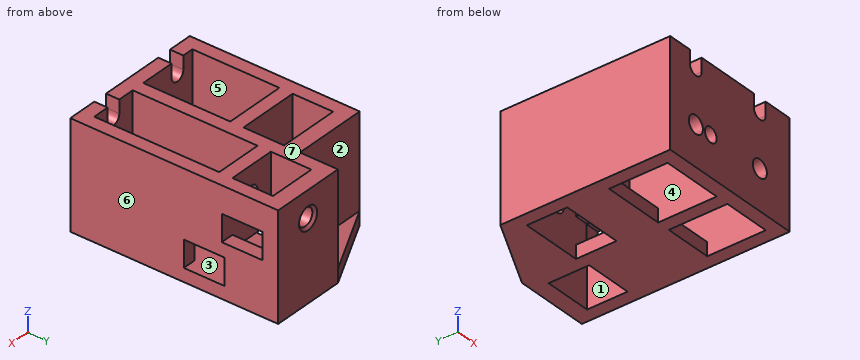
from build123d import *

# Parameters (mm, degrees)
SKETCH1_W           = 23
SKETCH1_H           = 32.75
SKETCH1_W_2         = 18
SKETCH1_H_2         = 15.25
SKETCH1_H_3         = 47.05
BOSS_EXTRUDE1_DEPTH = 40
CUT_EXTRUDE1_REACH  = 106.244
SKETCH2_R           = 2.75
CUT_EXTRUDE2_REACH  = 106.244
SKETCH3_W           = 10
SKETCH3_H           = 15.25
SKETCH4_W           = 10
SKETCH4_H           = 15.25
CUT_EXTRUDE3_DEPTH  = 102.645904984
CUT_EXTRUDE4_REACH  = 106.244
SKETCH6_R           = 3.25
CHAMFER1_SIZE       = 1
CUT_EXTRUDE5_REACH  = 106.244
SKETCH7_R           = 3.3
SKETCH9_R           = 2.75
CUT_EXTRUDE6_DEPTH  = 101.542975886
SKETCH10_W          = 18
SKETCH10_H          = 25
SKETCH10_W_2        = 23
SKETCH10_H_2        = 10.7
BOSS_EXTRUDE2_DEPTH = 5


with BuildPart() as part:
    # Sketch1 → Boss-Extrude1 (new body)
    with BuildSketch(Plane.XY):
        Polygon((0, 0), (0, 64), (28, 64), (28, 78.3), (56, 78.3), (56, 0), align=None)
        with Locations((16.5, 21.375)):
            Rectangle(SKETCH1_W, SKETCH1_H, mode=Mode.SUBTRACT)
        with Locations((42, 64.675)):
            Rectangle(SKETCH1_W_2, SKETCH1_H_2, mode=Mode.SUBTRACT)
        with Locations((16.5, 50.375)):
            Rectangle(SKETCH1_W, SKETCH1_H_2, mode=Mode.SUBTRACT)
        with Locations((42, 28.525)):
            Rectangle(SKETCH1_W_2, SKETCH1_H_3, mode=Mode.SUBTRACT)
    extrude(amount=BOSS_EXTRUDE1_DEPTH)

    # Cut-Extrude1: up to this face of the body (flat: up to its plane)
    cut_extrude1_end = Plane(part.part.faces().sort_by_distance((16.5, 37.75, 20))[0])
    # Sketch2 → Cut-Extrude1 (cut, up to the picked face)
    with BuildSketch(Plane(origin=(0, 78.3, 0), x_dir=(1, 0, 0), z_dir=(0, 1, 0)), mode=Mode.PRIVATE) as cut_extrude1_sk1:
        with Locations(Location((19, -15, 0), (0, 0, 270))):
            Circle(SKETCH2_R)
    cut_extrude1_tool1 = split(extrude(cut_extrude1_sk1.sketch, amount=-CUT_EXTRUDE1_REACH, mode=Mode.PRIVATE), bisect_by=cut_extrude1_end, keep=Keep.BOTH, mode=Mode.PRIVATE)
    # Sketch2 → Cut-Extrude1 (cut, up to the picked face)
    with BuildSketch(Plane(origin=(0, 78.3, 0), x_dir=(1, 0, 0), z_dir=(0, 1, 0)), mode=Mode.PRIVATE) as cut_extrude1_sk2:
        with Locations(Location((42, -30, 0), (0, 0, 270))):
            Circle(SKETCH2_R)
    cut_extrude1_tool2 = split(extrude(cut_extrude1_sk2.sketch, amount=-CUT_EXTRUDE1_REACH, mode=Mode.PRIVATE), bisect_by=cut_extrude1_end, keep=Keep.BOTH, mode=Mode.PRIVATE)
    add(cut_extrude1_tool1.solids().sort_by(Axis((19, 78.3, 15), (0, -1, 0)))[0], mode=Mode.SUBTRACT)
    add(cut_extrude1_tool2.solids().sort_by(Axis((42, 78.3, 30), (0, -1, 0)))[0], mode=Mode.SUBTRACT)

    # Sketch3 → Cut-Extrude2 (cut, up to next)
    with BuildSketch(Plane(origin=(56, 0, 0), x_dir=(0, 0, -1), z_dir=(1, 0, 0)), mode=Mode.PRIVATE) as cut_extrude2_sk1:
        with Locations((-25, 64.675)):
            Rectangle(SKETCH3_W, SKETCH3_H)
    cut_extrude2_tool1 = extrude(cut_extrude2_sk1.sketch, amount=-CUT_EXTRUDE2_REACH, mode=Mode.PRIVATE) & part.part
    add(cut_extrude2_tool1.solids().sort_by_distance((56, 64.675, 25))[0], mode=Mode.SUBTRACT)

    # Sketch4 → Cut-Extrude3 (cut, through all)
    with BuildSketch(Plane(origin=(5, 0, 0), x_dir=(0, 0, -1), z_dir=(1, 0, 0))):
        with Locations((-10, 50.375)):
            Rectangle(SKETCH4_W, SKETCH4_H)
    extrude(amount=CUT_EXTRUDE3_DEPTH, mode=Mode.SUBTRACT)

    # Sketch6 → Cut-Extrude4 (cut, up to next)
    with BuildSketch(Plane(origin=(0, 78.3, 0), x_dir=(1, 0, 0), z_dir=(0, 1, 0)), mode=Mode.PRIVATE) as cut_extrude4_sk1:
        with Locations(Location((19, -15, 0), (0, 0, 270))):
            Circle(SKETCH6_R)
    cut_extrude4_tool1 = extrude(cut_extrude4_sk1.sketch, amount=-CUT_EXTRUDE4_REACH, mode=Mode.PRIVATE) & part.part
    # Sketch6 → Cut-Extrude4 (cut, up to next)
    with BuildSketch(Plane(origin=(0, 78.3, 0), x_dir=(1, 0, 0), z_dir=(0, 1, 0)), mode=Mode.PRIVATE) as cut_extrude4_sk2:
        with Locations(Location((42, -30, 0), (0, 0, 270))):
            Circle(SKETCH6_R)
    cut_extrude4_tool2 = extrude(cut_extrude4_sk2.sketch, amount=-CUT_EXTRUDE4_REACH, mode=Mode.PRIVATE) & part.part
    add(cut_extrude4_tool1.solids().sort_by_distance((19, 78.3, 15))[0], mode=Mode.SUBTRACT)
    add(cut_extrude4_tool2.solids().sort_by_distance((42, 78.3, 30))[0], mode=Mode.SUBTRACT)

    # Chamfer1
    chamfer1_edges = [part.edges().sort_by_distance(p)[0] for p in [
        (19, 64, 11.75),
        (42, 78.3, 26.75),
    ]]
    chamfer(chamfer1_edges, length=CHAMFER1_SIZE)

    # Sketch7 → Cut-Extrude5 (cut, up to next)
    with BuildSketch(Plane.XZ, mode=Mode.PRIVATE) as cut_extrude5_sk1:
        with Locations((12, 15)):
            Circle(SKETCH7_R)
    cut_extrude5_tool1 = extrude(cut_extrude5_sk1.sketch, amount=-CUT_EXTRUDE5_REACH, mode=Mode.PRIVATE) & part.part
    # Sketch7 → Cut-Extrude5 (cut, up to next)
    with BuildSketch(Plane.XZ, mode=Mode.PRIVATE) as cut_extrude5_sk2:
        with Locations((42, 15)):
            Circle(SKETCH7_R)
    cut_extrude5_tool2 = extrude(cut_extrude5_sk2.sketch, amount=-CUT_EXTRUDE5_REACH, mode=Mode.PRIVATE) & part.part
    # Sketch7 → Cut-Extrude5 (cut, up to next)
    with BuildSketch(Plane.XZ, mode=Mode.PRIVATE) as cut_extrude5_sk3:
        with BuildLine():
            Line((9.25, 35), (9.25, 40))
            Line((9.25, 40), (14.75, 40))
            Line((14.75, 40), (14.75, 35))
            ThreePointArc((14.75, 35), (12, 32.25), (9.25, 35))
        make_face()
    cut_extrude5_tool3 = extrude(cut_extrude5_sk3.sketch, amount=-CUT_EXTRUDE5_REACH, mode=Mode.PRIVATE) & part.part
    # Sketch7 → Cut-Extrude5 (cut, up to next)
    with BuildSketch(Plane.XZ, mode=Mode.PRIVATE) as cut_extrude5_sk4:
        with BuildLine():
            Line((39.25, 35), (39.25, 40))
            Line((39.25, 40), (44.75, 40))
            Line((44.75, 40), (44.75, 35))
            ThreePointArc((44.75, 35), (42, 32.25), (39.25, 35))
        make_face()
    cut_extrude5_tool4 = extrude(cut_extrude5_sk4.sketch, amount=-CUT_EXTRUDE5_REACH, mode=Mode.PRIVATE) & part.part
    add(cut_extrude5_tool1.solids().sort_by_distance((12, 0, 15))[0], mode=Mode.SUBTRACT)
    add(cut_extrude5_tool2.solids().sort_by_distance((42, 0, 15))[0], mode=Mode.SUBTRACT)
    add(cut_extrude5_tool3.solids().sort_by_distance((12, 0, 36.393769))[0], mode=Mode.SUBTRACT)
    add(cut_extrude5_tool4.solids().sort_by_distance((42, 0, 36.393769))[0], mode=Mode.SUBTRACT)

    # Sketch9 → Cut-Extrude6 (cut, through all)
    with BuildSketch(Plane(origin=(0, 5, 0), x_dir=(1, 0, 0), z_dir=(0, 1, 0))):
        with Locations(Location((19, -15, 0), (0, 0, 270))):
            Circle(SKETCH9_R)
    extrude(amount=-CUT_EXTRUDE6_DEPTH, mode=Mode.SUBTRACT)

    # Sketch10 → Boss-Extrude2 (add)
    with BuildSketch(Plane(origin=(0, 0, 0), x_dir=(-1, 0, 0), z_dir=(0, 0, -1))):
        Polygon((-28, 78.3), (0, 64), (-28, 64), align=None)
        with Locations((-42, 39.55)):
            Rectangle(SKETCH10_W, SKETCH10_H)
        with Locations((-16.5, 32.4)):
            Rectangle(SKETCH10_W_2, SKETCH10_H_2)
    extrude(amount=-BOSS_EXTRUDE2_DEPTH)


solid = part.part
For this review, take the finished solid that the model builds, in its own axes (mm). Face numbers are marked on the shaded views. A direction names the side the tool comes from. Give positions to 0.01 mm unless a question says otherwise; leave off trailing zeros. Loops run counter-clockwise (first coordinate to the right, second up) from the corner with the lowest first, then second, coordinate; pieces in that order, holes last.
Item 1: Take a section at B-B, the plane y = 23.5. State the section outline as (x, z) points.
Item 2: Take a section at D-D, the plane x = 29. State the section outline as (y, z) points.
Item 3: Draft analysis for pull direction X (two halves, no side actions). For the marked faces 5, 6 and 7, state which applies: +X half, -X half, draft (parallel to the pull), parting line (faces both ways), or undercut.
Item 4: Take a section at C-C, the plane x = 42. Give the number of separate pieces and of enclosed holes in the cut face, and give its area (3 significant figures).
Item 5: For line 1 along Y through (x, z) = (47, 4); line 2 along X through (y, z) = (26, 20); line 3 along Y through (x, z) = (8, 33.5), list the stretches that pass through material, from the lowest coordinate up.
Item 6: Take a section at A-A, the plane x = 36. State the section outline as (y, z) points, and give its area (3 significant figures).
Item 7: Tool access review of the marked faces 1, 2, 3 and 4: name each direction out of +Z, -Z, +X, -X, +Y, -Y from which nothing blocks a thin tool from reaching the whole face with its end or side.
Item 8: Insertion check: pin 1 (4.5 mm diameter, centred on x = 19.5, y = 71, fed in from +Z); pin 2 (1.5 mm diameter, centred on x = 45.5, y = 59, fed in from +Z); pin 3 (6 mm diameter, centred on x = 42, z = 15, fed in from -Y); pin 4 (8.5 mm diameter, centred on x = 20, z = 22.5, fed in from +Y). Each pin has a flat end and moves straight along its axis. Give the tip position at first contact, or say it passes through.
Calculated:
1. outline: (0, 0) - (5, 0) - (5, 40) - (0, 40) - close; (28, 0) - (33, 0) - (33, 40) - (28, 40) - close; (51, 0) - (56, 0) - (56, 40) - (51, 40) - close
2. outline: (0, 0) - (78.3, 0) - (78.3, 40) - (0, 40) - close; hole (42.75, 5) - (58, 5) - (58, 15) - (42.75, 15) - close
3. face 5: undercut
3. face 6: +X half
3. face 7: draft
4. separate pieces: 7
4. enclosed holes: 0
4. area: 576 mm2
5. line 1: y = 0 to 5, 27.05 to 57.05, 72.3 to 78.3
5. line 2: x = 0 to 5, 28 to 33, 51 to 56
5. line 3: y = 0 to 5, 37.75 to 42.75, 58 to 64
6. outline: (0, 0) - (5, 0) - (5, 40) - (0, 40) - close; (27.05, 0) - (57.05, 0) - (57.05, 5) - (27.05, 5) - close; (52.05, 15) - (57.05, 15) - (57.05, 40) - (52.05, 40) - close; (72.3, 0) - (78.3, 0) - (78.3, 40) - (72.3, 40) - close
6. area: 715 mm2
7. face 1: +Z, -Z
7. face 2: +Z, -X, +Y
7. face 3: none
7. face 4: +Z
8. pin 1: stops at z = 5
8. pin 2: passes through
8. pin 3: stops at y = 52.05
8. pin 4: stops at y = 64
